Geometry check sheet. Reference: the model listing, model coordinates, mm. Face numbers are marked on the shaded views. A direction names the side the tool comes from. Round coordinates to 2 decimals unless told otherwise and drop trailing zeros. Write each loop counter-clockwise with the first axis right and the second up, starting at its lowest first coordinate (ties: lowest second). Pieces come first, ordered by that corner, then holes. Notation, with made-up numbers: (79, 83) -> (109, 83) arc R24 cw to (109, 118) -> close; hole circle Ø1 at (26.25, -1.5). An arc over 180 degrees is marked (long way). Return JSON: item names as keys, results as strings. Group by question number.
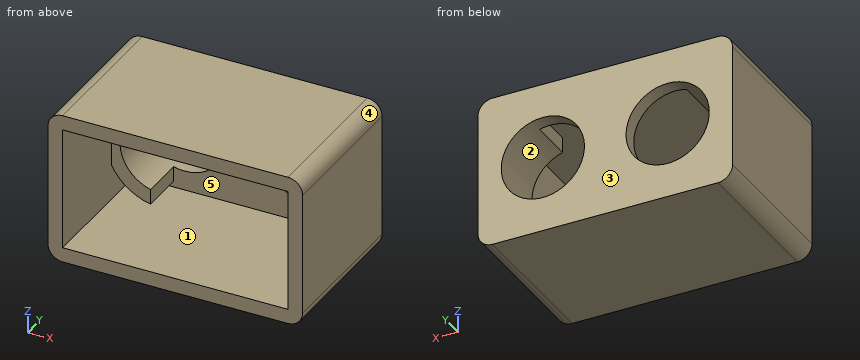
from build123d import *

# Parameters (mm, degrees)
CROQUIS1_W              = 52
CROQUIS1_H              = 31
CROQUIS1_W_2            = 46
CROQUIS1_H_2            = 25
SALIENTE_EXTRUIR1_DEPTH = 31
CROQUIS2_R              = 8.5
CORTAR_EXTRUIR1_DEPTH   = 31
REDONDEO1_R             = 3
VACIADO1_DEPTH          = 28
CROQUIS3_W              = 46
CROQUIS3_H              = 25
CORTAR_EXTRUIR2_DEPTH   = 19
CROQUIS4_W              = 30
CROQUIS4_H              = 23
CORTAR_EXTRUIR3_DEPTH   = 9


# Read off the part's stored shape, not the designer's step: Vaciado1
with BuildPart() as part:
    # Croquis1 → Saliente-Extruir1 (new body)
    # profile 1 of 2: a face of its own
    with BuildSketch(Plane(origin=(0, 0, 0), x_dir=(1, 0, 0), z_dir=(0, 1, 0))):
        Rectangle(CROQUIS1_W, CROQUIS1_H)
        Rectangle(CROQUIS1_W_2, CROQUIS1_H_2, mode=Mode.SUBTRACT)
    # profile 2 of 2: a face of its own
    with BuildSketch(Plane(origin=(0, 0, 0), x_dir=(1, 0, 0), z_dir=(0, 1, 0))):
        Rectangle(CROQUIS1_W_2, CROQUIS1_H_2)
    extrude(amount=SALIENTE_EXTRUIR1_DEPTH)

    # Croquis2 → Cortar-Extruir1 (cut)
    with BuildSketch(Plane(origin=(0, 31, 0), x_dir=(1, 0, 0), z_dir=(0, 1, 0))):
        with Locations(Location((-12.75, 0, 0), (0, 0, 270))):
            Circle(CROQUIS2_R)
        with Locations(Location((12.75, 0, 0), (0, 0, 270))):
            Circle(CROQUIS2_R)
    extrude(amount=-CORTAR_EXTRUIR1_DEPTH, mode=Mode.SUBTRACT)

    # Redondeo1
    redondeo1_edges = [part.edges().sort_by_distance(p)[0] for p in [
        (26, 15.5, 15.5),
        (-26, 15.5, 15.5),
        (-26, 15.5, -15.5),
        (26, 15.5, -15.5),
    ]]
    fillet(redondeo1_edges, radius=REDONDEO1_R)

    # Vaciado1 outline → Vaciado1 (cut)
    with BuildSketch(Plane(origin=(0, 0, 0), x_dir=(1, 0, 0), z_dir=(0, 1, 0))):
        with BuildLine():
            Line((-23, 12.5), (-23, 5.214163404))
            ThreePointArc((-23, 5.214163404), (-1.25, 0), (-23, -5.214163404))
            Line((-23, -5.214163404), (-23, -12.5))
            Line((-23, -12.5), (23, -12.5))
            Line((23, -12.5), (23, -5.214163404))
            ThreePointArc((23, -5.214163404), (1.25, 0), (23, 5.214163404))
            Line((23, 5.214163404), (23, 12.5))
            Line((23, 12.5), (-23, 12.5))
        make_face()
    extrude(amount=VACIADO1_DEPTH, mode=Mode.SUBTRACT)

    # Croquis3 → Cortar-Extruir2 (cut)
    with BuildSketch(Plane.XZ):
        Rectangle(CROQUIS3_W, CROQUIS3_H)
    extrude(amount=-CORTAR_EXTRUIR2_DEPTH, mode=Mode.SUBTRACT)

    # Croquis4 → Cortar-Extruir3 (cut)
    with BuildSketch(Plane.XZ.offset(-19)):
        Rectangle(CROQUIS4_W, CROQUIS4_H)
    extrude(amount=-CORTAR_EXTRUIR3_DEPTH, mode=Mode.SUBTRACT)


solid = part.part
1) Sectioned sample at C-C on x = -12.75. Enter the section's corners in (y, z), and give its area (3 significant figures).
2) Mould release check, pull along Z, two halves, no side actions. Record for the marked faces 3, 4 and 5: +Z half, -Z half, draft (parallel to the pull), parting line (faces both ways), or undercut.
3) Sectioned sample at B-B on y = 20.5. Enter the section's corners in (x, z).
4) Sectioned sample at A-A on z = 0. Enter the section's corners in (x, y), and give its area (4 significant figures).
5) Material ranges on probe 1 along Z at (x, y) = (9.5, 18.5); probe 2 along X at (y, z) = (7, -3.5); probe 3 along X at (y, z) = (24, 0), recorded low to high. Write a range as [from, to].
6) Sectioned sample at D-D on y = 29.5. Enter the section's corners in (x, z).
7) Go/stop test with flat-tipped pins: P1, Ø6.5, axis at x = 20.5, z = 5.5, coming from the -Y side; P2, Ø4, axis at x = -19, z = 3, coming from the -Y side; P3, Ø15.5, axis at x = -12.75, z = 0, coming from the +Y side (1 decimal). Record where each tip stops, or that it passes through.
8) Tool access check on the marked faces 1 and 2. Record the directions out of +Z, -Z, +X, -X, +Y, -Y that give a thin tool (end or side, any length) a straight path to the whole face; none if there is none.
Evaluation:
{
 "1": {"outline": "(0, -15.5) -> (31, -15.5) -> (31, -8.5) -> (28, -8.5) -> (28, -12.5) -> (0, -12.5) -> close; (0, 12.5) -> (28, 12.5) -> (28, 8.5) -> (31, 8.5) -> (31, 15.5) -> (0, 15.5) -> close", "area": "210 mm2"},
 "2": {"face 3": "draft", "face 4": "+Z half", "face 5": "undercut"},
 "3": {"outline": "(-26, -12.5) arc R3 ccw to (-23, -15.5) -> (23, -15.5) arc R3 ccw to (26, -12.5) -> (26, 12.5) arc R3 ccw to (23, 15.5) -> (-23, 15.5) arc R3 ccw to (-26, 12.5) -> close; hole (-23, -12.5) -> (23, -12.5) -> (23, -5.21) arc R11.5 cw to (15, -11.28) -> (15, -8.2) arc R8.5 ccw to (15, 8.2) -> (15, 11.28) arc R11.5 cw to (23, 5.21) -> (23, 12.5) -> (-23, 12.5) -> (-23, 5.21) arc R11.5 cw to (-15, 11.28) -> (-15, 8.2) arc R8.5 ccw to (-15, -8.2) -> (-15, -11.28) arc R11.5 cw to (-23, -5.21) -> close"},
 "4": {"outline": "(-26, 0) -> (-23, 0) -> (-23, 19) -> (-21.25, 19) -> (-21.25, 31) -> (-26, 31) -> close; (-4.25, 28) -> (4.25, 28) -> (4.25, 31) -> (-4.25, 31) -> close; (21.25, 19) -> (23, 19) -> (23, 0) -> (26, 0) -> (26, 31) -> (21.25, 31) -> close", "area": "253.5 mm2"},
 "5": {"probe 1": "z = [-15.5, -12.5], [12.5, 15.5]", "probe 2": "x = [-26, -23], [23, 26]", "probe 3": "x = [-26, -21.25], [21.25, 26]"},
 "6": {"outline": "(-26, -12.5) arc R3 ccw to (-23, -15.5) -> (23, -15.5) arc R3 ccw to (26, -12.5) -> (26, 12.5) arc R3 ccw to (23, 15.5) -> (-23, 15.5) arc R3 ccw to (-26, 12.5) -> close; hole circle Ø17 at (-12.75, 0); hole circle Ø17 at (12.75, 0)"},
 "7": {"P1": "stops at y = 0", "P2": "stops at y = 19", "P3": "passes through"},
 "8": {"face 1": "-Y", "face 2": "+Y, -Y"}
}
